from build123d import *

# Parameters (mm, degrees)
F0_W     = 400
F0_H     = 350
F1_DEPTH = 19
F4_DEPTH = 19.001
F2_R     = 20
F5_DEPTH = 12.5
F6_DEPTH = 19.0010001


with BuildPart() as f1:
    # F0 (on Top) → F1 (new body)
    with BuildSketch(Plane.XY):
        Rectangle(F0_W, F0_H)
    extrude(amount=F1_DEPTH)

    # F3 (on face) → F4 (cut, through all)
    with BuildSketch(Plane.XY.offset(19)):
        with BuildLine():
            add(Edge.make_bspline(
                [(151.2464284897, -175), (164.2430137507, -171.5517342548), (191.0711310333, -164.4336739354), (196.9625921733, -134.8047557028), (200, -119.5292398334)],
                knots=[0, 0, 0, 0, 0.484438961, 1, 1, 1, 1], degree=3))
            Line((151.2464284897, -175), (200, -175))
            Line((200, -175), (200, -119.5292398334))
        make_face()
    extrude(amount=-F4_DEPTH, mode=Mode.SUBTRACT)

    # F2 (on face) → F5 (cut, symmetric)
    with BuildSketch(Plane.XY.offset(19)):
        with Locations((122.5676462054, 137.3537778854)):
            Circle(F2_R)
        with Locations((33.6000025272, 137.3537778854)):
            Circle(F2_R)
        with Locations((-43.9001172781, 137.3537778854)):
            Circle(F2_R)
        with Locations((-123.9853724837, 137.3537778854)):
            Circle(F2_R)
    extrude(amount=F5_DEPTH, both=True, mode=Mode.SUBTRACT)

    # F2 (on face) → F6 (cut, through all)
    with BuildSketch(Plane.XY.offset(19)):
        with BuildLine():
            add(Edge.make_bspline(
                [(-157.191619277, 175), (-167.0547662133, 173.6002362151), (-188.1240063271, 173.8063038374), (-199.1158279923, 132.3396944698), (-200, 134.5333755016)],
                knots=[0, 0, 0, 0, 0.4262547571, 0.869833783, 0.869833783, 0.869833783, 0.869833783], degree=3))
            Line((-157.191619277, 175), (-200, 175))
            Line((-200, 175), (-200, 137.3537778854))
            Line((-200, 137.3537778854), (-200, 134.5333755016))
        make_face()
    extrude(amount=-F6_DEPTH, mode=Mode.SUBTRACT)


solid = f1.part
Design review of the part built by this model. Coordinates are the model's own, in mm. A direction names the side the tool comes from. Give positions to 0.01 mm unless a question says otherwise; leave off trailing zeros. Loops run counter-clockwise (first coordinate to the right, second up) from the corner with the lowest first, then second, coordinate; pieces in that order, holes last. Notation, with made-up numbers: (2.25, 58) - (50.25, 58) arc R10 ccw to (50.25, 74) - close; hole circle Ø5 at (36, 28). An arc over 180 degrees is marked (long way). Use CSV: the item, a comma, the result in double quotes. Start each with the question number.
1. Add section B-B (z = 11.5). Count the separate pieces of the cut face and the enclosed holes in it, plus the area to 3 significant figures.
2. Add section C-C (x = -138.5). State the section outline as (y, z) points, plus the area to 3 significant figures.
3. Machinability: for faces 1 (the flat face through (-124, 138, 6.5)), 2 (the flat face through (-3, 2, 19)), which of the approach directions +Z, -Z, +X, -X, +Y, -Y give a long, thin tool a straight path to every point of the face, cutting with its end or side? Answer none if there is none.
4. Add section A-A (x = 31.5). State the section outline as (y, z) points.
5. Draft analysis for pull direction X (two halves, no side actions). For faces 3 (the flat face through (-200, -22, 9)), 4 (the flat face through (200, 26, 9)), 5 (the flat face through (-27, -175, 9)), 6 (the flat face through (33, 138, 6.5)), state which applies: released by +X, released by -X, zero draft, split by the parting line, or undercut.
6. Insertion check: P1, Ø12, axis at x = -40.5, y = 147, coming from the +Z side. The pin has a flat end and moves straight along its axis. Give the tip position at first contact, or say it passes through.
7. Wall thickness on L1, parallel to X at y = 140.5, z = 9; L2, parallel to X at y = 125, z = 13.25; L3, parallel to Y at x = -119, z = 14.75: over which ranges is each line inside the solid? List them lowest first.
Results found:
1,separate pieces,"1"
1,enclosed holes,"4"
1,area,"134,000 mm²"
2,outline,"(-175, 0) - (175, 0) - (175, 19) - (151.11, 19) - (151.11, 6.5) - (123.59, 6.5) - (123.59, 19) - (-175, 19) - close"
2,area,"6,310 mm²"
3,face 1,"+Z"
3,face 2,"+Z, +X, -X, +Y, -Y"
4,outline,"(-175, 0) - (175, 0) - (175, 19) - (157.24, 19) - (157.24, 6.5) - (117.46, 6.5) - (117.46, 19) - (-175, 19) - close"
5,face 3,"released by -X"
5,face 4,"released by +X"
5,face 5,"zero draft"
5,face 6,"undercut"
6,P1,"stops at z = 6.5"
7,L1,"x = -196.97 to -143.74, -104.23 to -63.65, -24.15 to 13.85, 53.35 to 102.82, 142.32 to 200"
7,L2,"x = -200 to -139.71, -108.26 to -59.63, -28.17 to 17.87, 49.33 to 106.84, 138.3 to 200"
7,L3,"y = -175 to 117.99, 156.72 to 175"
